Build history of the part. All positions in model axes, mm. Give positions to 0.01 mm unless a question says otherwise; leave off trailing zeros. Write each loop counter-clockwise with the first axis right and the second up, starting at its lowest first coordinate (ties: lowest second). Pieces come first, ordered by that corner, then holes. Notation, with made-up numbers: M 58,67 L 117,67 A21 cw 117,104 Z; hole C 0.25,9.25 d5. An arc over 180 degrees is marked long. Return JSON: item names as keys, results as strings. Group by question number.
Q1. Flat gauge pin, fed straight in: pin 1 Ø2 at (x, y) = (-99.5, 1.5) entering from -Z. Where does the tip first touch, or does it go through?
Q2. Wall check: probe 1 along X at (y, z) = (3.8, 6.5); probe 2 along X at (y, z) = (1.85, 4.25); probe 3 along Z at (x, y) = (-121, 0.4). Give the ranges that are in metal, low to high.
Q3. Band-saw the part on C-C, the plane z = 5.5. Give the cut face in (x, y), then the cut area to 3 significant figures.
Q4. Band-saw the part on A-A, the plane y = 1.15. Give the cut face in (x, z).
Q5. Band-saw the part on B-B, the plane z = -6.75. Give the cut face in (x, y).
from build123d import *

# Parameters (mm, degrees)
ESQUISSE1_W             = 270
ESQUISSE1_H             = 23
BOSS_EXTRU_1_DEPTH      = 5
ENL_V_MAT_EXTRU_1_DEPTH = 10
ENL_V_MAT_EXTRU_2_DEPTH = 10


with BuildPart() as part:
    # Esquisse1 → Boss.-Extru.1 (new body)
    with BuildSketch(Plane(origin=(0, 0, 0), x_dir=(1, 0, 0), z_dir=(0, 1, 0))):
        Rectangle(ESQUISSE1_W, ESQUISSE1_H)
    extrude(amount=BOSS_EXTRU_1_DEPTH)

    # Esquisse3 → Enlèv. mat.-Extru.1 (cut)
    with BuildSketch(Plane(origin=(0, 5, 0), x_dir=(1, 0, 0), z_dir=(0, 1, 0))):
        Polygon((135, -8.5), (135, 11.5), (95, 11.5), align=None)
    extrude(amount=-ENL_V_MAT_EXTRU_1_DEPTH, mode=Mode.SUBTRACT)

    # Esquisse5 → Enlèv. mat.-Extru.2 (cut)
    with BuildSketch(Plane(origin=(0, 5, 0), x_dir=(1, 0, 0), z_dir=(0, 1, 0))):
        Polygon((-135, 11.5), (-95, 11.5), (-135, -8.5), align=None)
    extrude(amount=-ENL_V_MAT_EXTRU_2_DEPTH, mode=Mode.SUBTRACT)


solid = part.part
From the geometry:
{
 "1": {"pin 1": "stops at z = -9.75"},
 "2": {"probe 1": "x = -131 to 131", "probe 2": "x = -126.5 to 126.5", "probe 3": "z = 1.5 to 11.5"},
 "3": {"outline": "M -129,0 L 129,0 L 129,5 L -129,5 Z", "area": "1,290 mm^2"},
 "4": {"outline": "M -135,8.5 L -95,-11.5 L 95,-11.5 L 135,8.5 L 135,11.5 L -135,11.5 Z"},
 "5": {"outline": "M -104.5,0 L 104.5,0 L 104.5,5 L -104.5,5 Z"}
}
